Study the drawing (mm; zero at the part's minimum x, y, z) and answer. Give positions to 0.01 mm unless a question says otherwise; leave off trailing zeros. Order: outer loops, then holes, each group sorted by start corner. A loop starts at its lowest first (then second) coordinate and runs counter-clockwise, first axis right, second up. Notation, with made-up numbers: (5.5, 13) -> (27.5, 13) arc R26 ccw to (27.5, 51) -> close; hole circle Ø11 at (-19, 55). An arc over 180 degrees is marked (long way). One line per question, with ' | ' between items. Start each with the question number.
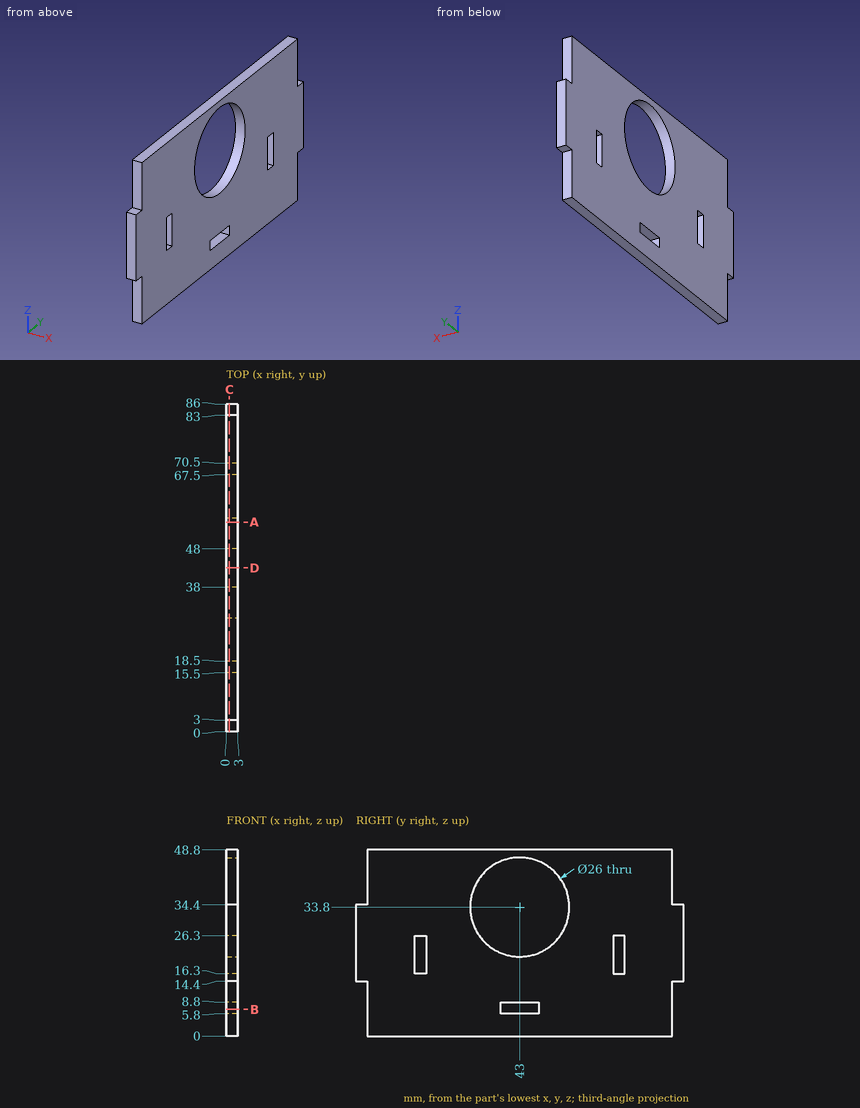
Q1. Given P1, Ø1.5, axis at x = 1, z = 44.5, coming from the -Y side; P2, Ø1, axis at x = 2, z = 35.5, coming from the +Y side; P3, Ø0.9, axis at x = 1, y = 85, coming from the +Z side; P4, Ø1.5, axis at x = 1, y = 25.5, coming from the -Z side, each flat-ended and moving along its own axis, determine where each tip first touches the part or whether it passes through.
Q2. A cutting plane is placed at A-A, the plane y = 55. Determine the outline of the cut face in (x, z), then the cut area to 3 significant figures.
Q3. A cutting plane is placed at D-D, the plane y = 43. Determine the outline of the cut face in (x, z), then the cut area to 3 significant figures.
Q4. A cutting plane is placed at B-B, the plane z = 7. Determine the outline of the cut face in (x, y).
Q5. Find the intervals of material crossed by line 1 (Z direction, x = 2.3, y = 43); line 2 (Y direction, x = 0.8, z = 20.5); line 3 (Y direction, x = 1.6, z = 4), in increasing order.
Q6. A cutting plane is placed at C-C, the plane x = 0.8. Determine the outline of the cut face in (y, z).
Geometry results:
1) P1: y = 3 | P2: y = 83 | P3: z = 34.4 | P4: z = 0
2) outline: (0, 0) -> (3, 0) -> (3, 28.8) -> (0, 28.8) -> close; (0, 38.8) -> (3, 38.8) -> (3, 48.8) -> (0, 48.8) -> close | area: 116 mm²
3) outline: (0, 0) -> (3, 0) -> (3, 5.8) -> (0, 5.8) -> close; (0, 8.8) -> (3, 8.8) -> (3, 20.8) -> (0, 20.8) -> close; (0, 46.8) -> (3, 46.8) -> (3, 48.8) -> (0, 48.8) -> close | area: 59.4 mm²
4) outline: (0, 3) -> (3, 3) -> (3, 38) -> (0, 38) -> close; (0, 48) -> (3, 48) -> (3, 83) -> (0, 83) -> close
5) line 1: 0 to 5.8, 8.8 to 20.8, 46.8 to 48.8 | line 2: 0 to 15.5, 18.5 to 67.5, 70.5 to 86 | line 3: 3 to 83
6) outline: (0, 14.4) -> (3, 14.4) -> (3, 0) -> (83, 0) -> (83, 14.4) -> (86, 14.4) -> (86, 34.4) -> (83, 34.4) -> (83, 48.8) -> (3, 48.8) -> (3, 34.4) -> (0, 34.4) -> close; hole (15.5, 16.3) -> (18.5, 16.3) -> (18.5, 26.3) -> (15.5, 26.3) -> close; hole circle Ø26 at (43, 33.8); hole (38, 5.8) -> (48, 5.8) -> (48, 8.8) -> (38, 8.8) -> close; hole (67.5, 16.3) -> (70.5, 16.3) -> (70.5, 26.3) -> (67.5, 26.3) -> close
